Autodesk Inventor part; units mm, degrees
ref_plane "YZ Plane" through (0, 0, 0) normal (1, 0, 0) x (0, 1, 0)
ref_plane "XZ Plane" through (0, 0, 0) normal (0, 1, 0) x (-1, 0, 0)
ref_plane "XY Plane" through (0, 0, 0) normal (0, 0, 1) x (1, 0, 0)
sketch "Sketch1" plane through (0, 0, 0) normal (0, 1, 0) x (-1, 0, 0)
  line L0 (0, 0) -> (42, 0)
  circle A0 centre (42, 0) radius 3
  circle A1 centre (0, 0) radius 3
  line L1 (0, 0) -> (-8, 0)
  line L2 (-8, 0) -> (-8, -8)
  line L3 (42, 0) -> (42, 8)
  line L4 (42, 8) -> (50, 8)
  line L5 (50, 8) -> (-8, 8)
  line L6 (-8, 8) -> (-8, -8)
  line L7 (-8, -8) -> (50, -8)
  line L8 (50, -8) -> (50, 8)
  dimension "d0" = 42
  dimension "d1" = 6
  dimension "d2" = 6
  dimension "d3" = 8
  dimension "d4" = 8
  dimension "d5" = 8
  dimension "d6" = 8
extrude "Extrusion1" add sketch "Sketch1" along normal blind 24 contours A1 L1 L6 L5 L3 A0 L0 | L0 A0 L3 L4 L8 L7 L2 L1 A1
fillet "Fillet1" radius 2 4 edges at (8, 12, 8) (8, 12, -8) (-50, 12, 8) (-50, 12, -8)
properties part number "Bearing Seat 8mm"
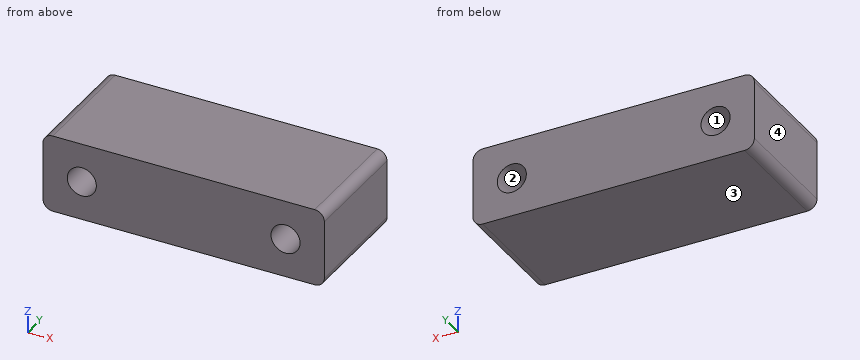
Can you work these out from the model? Positions are in its coordinate system, mm. Face numbers are marked on the shaded views. Round coordinates to 2 decimals unless told otherwise and drop trailing zeros. Order: outer loops, then holes, each group sorted by start corner. A loop starts at its lowest first (then second) coordinate and runs counter-clockwise, first axis right, second up. Notation, with made-up numbers: (7.25, 4) - (44.25, 4) arc R34 ccw to (44.25, 40) - close; hole circle Ø8 at (25, 77). An arc over 180 degrees is marked (long way). Answer in a Markdown table with one row per item.
(1) Suppose I cut it at A-A, the plane x = 0. Please give me the cut outline in (y, z), plus the area to 3 significant figures.
From the geometry:
| item | result |
|---|---|
| outline | (0, -8) - (24, -8) - (24, -3) - (0, -3) - close; (0, 3) - (24, 3) - (24, 8) - (0, 8) - close |
| area | 240 mm2 |
(2) If we mould it in two halves opening along Z, with no side actions, what happens to the marked faces 1, 2, 3 and 4? For each: released by +Z, released by -Z, zero draft, split by the parting line, or undercut.
From the geometry:
| item | result |
|---|---|
| face 1 | undercut |
| face 2 | undercut |
| face 3 | released by -Z |
| face 4 | zero draft |
(3) Suppose I cut it at C-C, the plane y = 6. Please give me the cut outline in (x, z).
From the geometry:
| item | result |
|---|---|
| outline | (-50, -6) arc R2 ccw to (-48, -8) - (6, -8) arc R2 ccw to (8, -6) - (8, 6) arc R2 ccw to (6, 8) - (-48, 8) arc R2 ccw to (-50, 6) - close; hole circle Ø6 at (-42, 0); hole circle Ø6 at (0, 0) |
(4) For P1, Ø3.5, axis at x = -42, z = 0, coming from the +Y side, with a flat end and sliding along its axis, tell me the tip position at first contact or that it passes through.
From the geometry:
| item | result |
|---|---|
| P1 | passes through |
(5) Suppose I cut it at B-B, the plane z = 0. Please give me the cut outline in (x, y), plus the area to 3 significant figures.
From the geometry:
| item | result |
|---|---|
| outline | (-50, 0) - (-45, 0) - (-45, 24) - (-50, 24) - close; (-39, 0) - (-3, 0) - (-3, 24) - (-39, 24) - close; (3, 0) - (8, 0) - (8, 24) - (3, 24) - close |
| area | 1,100 mm2 |
(6) Please list where these lines run through material, in increasing order: L1, parallel to X at y = 7.25, z = 0; L2, parallel to X at y = 22.25, z = 2.5; L3, parallel to Z at x = 0, y = 9.5. Write a range as from..to.
From the geometry:
| item | result |
|---|---|
| L1 | x = -50..-45, -39..-3, 3..8 |
| L2 | x = -50..-43.66, -40.34..-1.66, 1.66..8 |
| L3 | z = -8..-3, 3..8 |
